Could you check a few things on this model? Use its own coordinates, in mm. Give positions to 0.01 mm unless a question says otherwise; leave off trailing zeros. Write each loop counter-clockwise with the first axis right and the second up, starting at its lowest first coordinate (ties: lowest second). Pieces come first, ordered by that corner, then holes. Notation, with made-up numbers: (-12.5, 42) - (37.5, 42) arc R17 ccw to (37.5, 64) - close; hole circle Ø4 at (23, 0.25). An arc over 180 degrees is marked (long way). Answer as CSV lines item,"result". Start each with the question number.
Q1. Will this pin go through, and if not, where does the flat tip stop? pin 1 Ø5 at (x, y) = (-0.5, 6.5) entering from +Z.
Q2. Imagine slicing it at A-A on z = 1. List the corners of the cut face in (x, y) for me (3 decimals).
Q3. If I drill on line 1 along Y through (x, z) = (2, 0.4); line 2 along Y through (x, z) = (2.65, 0.55); line 3 along Y through (x, z) = (-5.75, 0.2), over which ranges is the centre line in solid material (lowest first)?
Q4. Imagine slicing it at B-B on y = 2.5. List the corners of the cut face in (x, z) for me, and give its area (3 significant figures).
Q5. Imagine slicing it at C-C on x = -4.5. List the corners of the cut face in (y, z) for me, and give its area (3 significant figures).
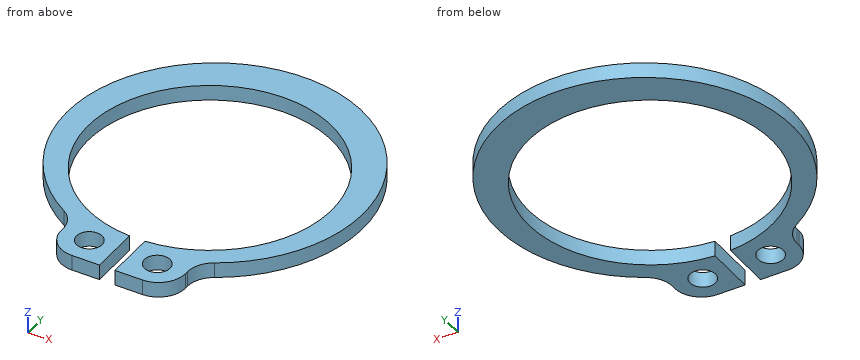
```python
from build123d import *

# Parameters (mm, degrees)
BOSS_EXTRUDE1_DEPTH = 1.2
SKETCH2_R           = 1
CUT_EXTRUDE1_DEPTH  = 18.715124188
FILLET1_R           = 2.1
FILLET2_R           = 2.1


with BuildPart() as part:
    # Sketch1 → Boss-Extrude1 (new body)
    with BuildSketch(Plane.XY):
        with BuildLine():
            Line((-4.85, -9.779813485), (-4.85, -13.4))
            Line((-4.85, -13.4), (-0.6, -13.4))
            Line((-0.6, -13.4), (-0.6, -9.481033699))
            ThreePointArc((-0.6, -9.481033699), (0, 9.5), (0.6, -9.481033699))
            Line((0.6, -9.481033699), (0.6, -13.4))
            Line((0.6, -13.4), (4.85, -13.4))
            Line((4.85, -13.4), (4.85, -9.779813485))
            ThreePointArc((4.85, -9.779813485), (0, 12.2), (-4.85, -9.779813485))
        make_face()
    extrude(amount=BOSS_EXTRUDE1_DEPTH)

    # Sketch2 → Cut-Extrude1 (cut, through all)
    with BuildSketch(Plane(origin=(0, 0, 0), x_dir=(-1, 0, 0), z_dir=(0, 0, -1))):
        with Locations((-2.65, -11.3)):
            Circle(SKETCH2_R)
        with Locations((2.65, -11.3)):
            Circle(SKETCH2_R)
    extrude(amount=-CUT_EXTRUDE1_DEPTH, mode=Mode.SUBTRACT)

    # Fillet1
    fillet1_edges = [part.edges().sort_by_distance(p)[0] for p in [
        (4.85, -9.779813485, 0.6),
        (-4.85, -9.779813485, 0.6),
    ]]
    fillet(fillet1_edges, radius=FILLET1_R)

    # Fillet2
    fillet2_edges = [part.edges().sort_by_distance(p)[0] for p in [
        (4.85, -13.4, 0.6),
        (-4.85, -13.4, 0.6),
    ]]
    fillet(fillet2_edges, radius=FILLET2_R)


solid = part.part
```
Conclusion:
1,pin 1,"through"
2,outline,"(-5.879, -9.238) arc R2.1 cw to (-4.85, -11.044) - (-4.85, -11.3) arc R2.1 ccw to (-2.75, -13.4) - (-0.6, -13.4) - (-0.6, -9.481) arc R9.5 cw (long way) to (0.6, -9.481) - (0.6, -13.4) - (2.75, -13.4) arc R2.1 ccw to (4.85, -11.3) - (4.85, -11.044) arc R2.1 cw to (5.879, -9.238) arc R11.525 ccw (long way) to start; hole circle Ø2 at (-2.65, -11.3); hole circle Ø2 at (2.65, -11.3)"
3,line 1,"-13.4 to -12.06, -10.54 to -9.29, 9.29 to 12.03"
3,line 2,"-13.4 to -12.3, -10.3 to -9.12, 9.12 to 11.89"
3,line 3,"-9.32 to -7.56, 7.56 to 10.66"
4,outline,"(-11.38, 0) - (-9.17, 0) - (-9.17, 1.2) - (-11.38, 1.2) - close; (9.17, 0) - (11.38, 0) - (11.38, 1.2) - (9.17, 1.2) - close"
4,area,"5.31 mm^2"
5,outline,"(-12.46, 0) - (-8.37, 0) - (-8.37, 1.2) - (-12.46, 1.2) - close; (8.37, 0) - (11.29, 0) - (11.29, 1.2) - (8.37, 1.2) - close"
5,area,"8.42 mm^2"
